from build123d import *

# Parameters (mm, degrees)
PAD_DEPTH    = 2.5
PAD001_DEPTH = 3
PAD002_DEPTH = 2.5
PAD003_DEPTH = 2.5
POCKET_DEPTH = 2.501


with BuildPart() as part:
    # Sketch → Pad (new body)
    with BuildSketch(Plane.XY):
        with BuildLine():
            ThreePointArc((-1.5, 3), (-4.5, 0), (-1.5, -3))
            Line((-1.5, -3), (1.5, -3))
            ThreePointArc((1.5, -3), (4.5, 0), (1.5, 3))
            Line((1.5, 3), (-1.5, 3))
        make_face()
    extrude(amount=PAD_DEPTH)

    # Sketch001 (on Face6 of Pad) → Pad001 (join)
    with BuildSketch(Plane.XY.offset(2.5)):
        with BuildLine():
            ThreePointArc((2, 1), (0, 3), (-2, 1))
            Line((-2, 1), (-2, -1))
            ThreePointArc((-2, -1), (0, -3), (2, -1))
            Line((2, -1), (2, 1))
        make_face()
    extrude(amount=PAD001_DEPTH)

    # Sketch002 (on Face12 of Pad001) → Pad002 (join)
    with BuildSketch(Plane.XY.offset(5.5)):
        with BuildLine():
            ThreePointArc((3, 40), (0, 43), (-3, 40))
            Line((-3, 40), (-3, 0))
            ThreePointArc((-3, 0), (0, -3), (3, 0))
            Line((3, 0), (3, 40))
        make_face()
    extrude(amount=PAD002_DEPTH)

    # Sketch003 (on Face17 of Pad002) → Pad003 (join)
    with BuildSketch(Plane.XY.offset(8)):
        with BuildLine():
            ThreePointArc((-3, 43), (-8, 38), (-3, 33))
            Line((-3, 33), (3, 33))
            ThreePointArc((3, 33), (8, 38), (3, 43))
            Line((-3, 43), (3, 43))
        make_face()
    extrude(amount=-PAD003_DEPTH)

    # Sketch004 (on Face15 of Pad003) → Pocket (cut, through all)
    with BuildSketch(Plane(origin=(0, 0, 5.5), x_dir=(1, 0, 0), z_dir=(0, 0, -1))):
        with BuildLine():
            ThreePointArc((-0.5, -35.4), (-3.1, -38), (-0.5, -40.6))
            Line((-0.5, -40.6), (0.5, -40.6))
            ThreePointArc((0.5, -40.6), (3.1, -38), (0.5, -35.4))
            Line((0.5, -35.4), (-0.5, -35.4))
        make_face()
    extrude(amount=-POCKET_DEPTH, mode=Mode.SUBTRACT)


solid = part.part
Geometry: final body of the model. Coordinates: model frame, mm. A direction names the side the tool comes from. Round coordinates to 2 decimals unless told otherwise and drop trailing zeros. Loops run counter-clockwise (first coordinate to the right, second up) from the corner with the lowest first, then second, coordinate; pieces in that order, holes last. Notation, with made-up numbers: (87.5, 75) - (105.5, 75) arc R16 ccw to (105.5, 91) - close; hole circle Ø11 at (-32, -3). An arc over 180 degrees is marked (long way). Write each question's results on one line, items separated by ' | '. Start each with the question number.
1) Cut plane C-C on x = 6. Return loops of the section in (y, z), then the cut area to 3 significant figures.
2) Cut plane A-A on z = 6.5. Return loops of the section in (x, y), then the cut area to 3 significant figures.
3) Mould query, pull axis X, two halves, no side actions, for faces 4 (the face through (-3.1, 37.9, 6.7)), 5 (the face through (2, 0, 4)), 6 (the face through (0, 43, 7)). Classes: released by +X, released by -X, zero draft, split by the parting line, or undercut.
4) Cut plane B-B on y = 38. Return loops of the section in (x, z), then the cut area to 3 significant figures.
5) Cut plane D-D on z = 4. Return loops of the section in (x, y), then the cut area to 3 significant figures.
6) Access query for faces 1 (the face through (0, -3, 7)), 2 (the face through (-4.5, 0.1, 1.2)), 3 (the face through (0, 40.6, 7)). Directions: +Z, -Z, +X, -X, +Y, -Y. A direction counts if a zero-diameter tool reaches every point of the face in a straight line with its end or side. Return the directions, or none.
7) First-contact query: P1, Ø0.8, axis at y = 11.5, z = 6.5, coming from the -X side; P2, Ø3, axis at x = -0.5, z = 1, coming from the +Y side; P3, Ø3, axis at y = 19.5, z = 6.5, coming from the +X side. Flat tips, straight axial feed; report the tip coordinate or a pass-through.
8) Line query: probe 1 along Z at (x, y) = (1.75, 13.5); probe 2 along X at (y, z) = (24, 6.5). Output: solid intervals per line, ascending. Write a range as [from, to].
Verdict:
1) outline: (34, 5.5) - (42, 5.5) - (42, 8) - (34, 8) - close | area: 20.0 mm2
2) outline: (-3, 0) arc R3 ccw to (3, 0) - (3, 33) arc R5 ccw to (3, 43) - (-3, 43) arc R5 ccw to (-3, 33) - close; hole (-0.5, 35.4) - (0.5, 35.4) arc R2.6 ccw to (0.5, 40.6) - (-0.5, 40.6) arc R2.6 ccw to start | area: 324 mm2
3) face 4: undercut | face 5: released by +X | face 6: zero draft
4) outline: (-8, 5.5) - (-3.1, 5.5) - (-3.1, 8) - (-8, 8) - close; (3.1, 5.5) - (8, 5.5) - (8, 8) - (3.1, 8) - close | area: 24.5 mm2
5) outline: (-2, -1) arc R2 ccw to (2, -1) - (2, 1) arc R2 ccw to (-2, 1) - close | area: 20.6 mm2
6) face 1: +Z, -Y | face 2: -Z, -X | face 3: +Z, -Z
7) P1: stops at x = -3 | P2: stops at y = 3 | P3: stops at x = 3
8) probe 1: z = [5.5, 8] | probe 2: x = [-3, 3]
